from build123d import *

# Parameters (mm, degrees)
BOSS_EXTRUDE1_DEPTH = 3.2
SKETCH3_R           = 3.25
SKETCH3_R_2         = 2.3
BOSS_EXTRUDE2_DEPTH = 1.3
FILLET1_R           = 3
FILLET2_R           = 1.5
FILLET3_R           = 1


with BuildPart() as part:
    # Sketch2 → Boss-Extrude1 (new body)
    with BuildSketch(Plane.XY):
        Polygon((-5.64375, 3.51875), (5.64375, 3.51875), (8.187159214, -5.552325228), (4.958101353, -6.457710236), (4.23125, -4.38125), (-4.23125, -4.38125), (-4.958101353, -6.457710236), (-8.187159214, -5.552325228), align=None)
    extrude(amount=BOSS_EXTRUDE1_DEPTH)

    # Sketch3 → Boss-Extrude2 (add)
    with BuildSketch(Plane.XY.offset(3.2)):
        with Locations((0, -0.43125)):
            Circle(SKETCH3_R)
        with Locations((0, -0.43125)):
            Circle(SKETCH3_R_2, mode=Mode.SUBTRACT)
    extrude(amount=BOSS_EXTRUDE2_DEPTH)

    # Fillet1
    fillet1_edges = [part.edges().sort_by_distance(p)[0] for p in [
        (-5.64375, 3.51875, 1.6),
        (5.64375, 3.51875, 1.6),
    ]]
    fillet(fillet1_edges, radius=FILLET1_R)

    # Fillet2
    fillet2_edges = [part.edges().sort_by_distance(p)[0] for p in [
        (8.187159214, -5.552325228, 1.6),
        (-8.187159214, -5.552325228, 1.6),
    ]]
    fillet(fillet2_edges, radius=FILLET2_R)

    # Fillet3
    fillet3_edges = [part.edges().sort_by_distance(p)[0] for p in [
        (4.958101353, -6.457710236, 1.6),
        (-4.958101353, -6.457710236, 1.6),
    ]]
    fillet(fillet3_edges, radius=FILLET3_R)


solid = part.part
Verification items for the finished model (mm, model axes). A direction names the side the tool comes from. Give positions to 0.01 mm unless a question says otherwise; leave off trailing zeros. Write each loop counter-clockwise with the first axis right and the second up, starting at its lowest first coordinate (ties: lowest second). Pieces come first, ordered by that corner, then holes.
(1) Cross-section at D-D (y = -2.5). Enter the section's corners in (x, z), plus the area to 3 significant figures.
(2) Access from +Z, -Z, +X, -X, +Y, -Y to the whole of each face (thin tool, end or side, straight path). Record for faces 1 (the face through (4.44, -4.98, 1.58)), 2 (the face through (6.31, -6.08, 1.58)), 3 (the face through (-2.58, -2.41, 3.84)).
(3) Mould release check, pull along X, two halves, no side actions. Record for faces 4 (the face through (7.01, -1.35, 1.58)), 5 (the face through (-0.499, -2.677, 3.841)), 6 (the face through (0, 0, 3.2)), 7 (the face through (-7.654, -5.233, 1.622)): +X half, -X half, draft (parallel to the pull), parting line (faces both ways), or undercut.
(4) Cross-section at B-B (y = -5). Enter the section's corners in (x, z).
(5) Cross-section at C-C (x = 0). Enter the section's corners in (y, z), plus the area to 4 significant figures.
(6) Gauge pin test, flat ends, axial feed: pin 1 (3.5 mm diameter, centred on x = 0.5, y = -0.5, fed in from +Z); pin 2 (1 mm diameter, centred on x = -1, z = 2, fed in from -Y). Record the tip position at first contact, or that the pin passes through.
(7) Material ranges on line 1 (Y direction, x = 0, z = 4.25); line 2 (Z direction, x = -0.25, y = 1.75); line 3 (X direction, y = -5, z = 2.8), recorded low to high.
(8) Cross-section at A-A (z = 1.1). Enter the section's corners in (x, y), plus the area to 3 significant figures.
Worked out:
1. outline: (-7.33, 0) - (7.33, 0) - (7.33, 3.2) - (2.51, 3.2) - (2.51, 4.5) - (1.01, 4.5) - (1.01, 3.2) - (-1.01, 3.2) - (-1.01, 4.5) - (-2.51, 4.5) - (-2.51, 3.2) - (-7.33, 3.2) - close
1. area: 50.8 mm2
2. face 1: +Z, -Z, -Y
2. face 2: +Z, -Z, +X, -Y
2. face 3: +Z
3. face 4: +X half
3. face 5: undercut
3. face 6: undercut
3. face 7: -X half
4. outline: (-7.76, 0) - (-4.45, 0) - (-4.45, 3.2) - (-7.76, 3.2) - close; (4.45, 0) - (7.76, 0) - (7.76, 3.2) - (4.45, 3.2) - close
5. outline: (-4.38, 0) - (3.52, 0) - (3.52, 3.2) - (2.82, 3.2) - (2.82, 4.5) - (1.87, 4.5) - (1.87, 3.2) - (-2.73, 3.2) - (-2.73, 4.5) - (-3.68, 4.5) - (-3.68, 3.2) - (-4.38, 3.2) - close
5. area: 27.75 mm2
6. pin 1: stops at z = 3.2
6. pin 2: stops at y = -4.38
7. line 1: y = -3.68 to -2.73, 1.87 to 2.82
7. line 2: z = 0 to 3.2
7. line 3: x = -7.76 to -4.45, 4.45 to 7.76
8. outline: (-7.78, -4.11) arc R1.5 ccw to (-6.74, -5.96) - (-5.86, -6.2) arc R1 ccw to (-4.65, -5.57) - (-4.23, -4.38) - (4.23, -4.38) - (4.65, -5.57) arc R1 ccw to (5.86, -6.2) - (6.74, -5.96) arc R1.5 ccw to (7.78, -4.11) - (6.26, 1.33) arc R3 ccw to (3.37, 3.52) - (-3.37, 3.52) arc R3 ccw to (-6.26, 1.33) - close
8. area: 115 mm2
